from build123d import *

# Parameters (mm, degrees)
F1_DEPTH  = 7.5
F3_DEPTH  = 6
F5_DEPTH  = 3
F7_DEPTH  = 5
F8_W      = 24
F8_H      = 1.5
F9_DEPTH  = 3.75
F10_W     = 19
F10_H     = 2.5
F11_DEPTH = 9.7
F12_R     = 0.75
F13_DEPTH = 7.7
F14_W     = 24
F14_H     = 1.5
F15_DEPTH = 3.75
F16_DEPTH = 9.7


with BuildPart() as f1:
    # F0 (on Top) → F1 (new body)
    with BuildSketch(Plane.XY):
        with BuildLine():
            Line((-19.5, -14.9), (19.5, -14.9))
            ThreePointArc((19.5, -14.9), (20.9142135624, -14.3142135624), (21.5, -12.9))
            Line((21.5, -12.9), (21.5, 12.9))
            ThreePointArc((21.5, 12.9), (20.9142135624, 14.3142135624), (19.5, 14.9))
            Line((19.5, 14.9), (-19.5, 14.9))
            ThreePointArc((-19.5, 14.9), (-20.9142135624, 14.3142135624), (-21.5, 12.9))
            Line((-21.5, 12.9), (-21.5, -12.9))
            ThreePointArc((-21.5, -12.9), (-20.9142135624, -14.3142135624), (-19.5, -14.9))
        make_face()
    extrude(amount=F1_DEPTH)

    # F2 (on Top) → F3 (cut)
    with BuildSketch(Plane.XY):
        with BuildLine():
            Line((-13, -9.2), (13, -9.2))
            Line((13, -9.2), (13, -12.9))
            Line((13, -12.9), (17.5, -12.9))
            ThreePointArc((17.5, -12.9), (18.9142135624, -12.3142135624), (19.5, -10.9))
            Line((19.5, -10.9), (19.5, -7.5))
            Line((19.5, -7.5), (17.25, -7.5))
            Line((17.25, -7.5), (17.25, 7.5))
            Line((17.25, 7.5), (19.5, 7.5))
            Line((19.5, 7.5), (19.5, 10.9))
            ThreePointArc((19.5, 10.9), (18.9142135624, 12.3142135624), (17.5, 12.9))
            Line((17.5, 12.9), (13, 12.9))
            Line((13, 12.9), (13, 9.2))
            Line((13, 9.2), (-13, 9.2))
            Line((-13, 9.2), (-13, 12.9))
            Line((-13, 12.9), (-17.5, 12.9))
            ThreePointArc((-17.5, 12.9), (-18.9142135624, 12.3142135624), (-19.5, 10.9))
            Line((-19.5, 10.9), (-19.5, 7.5))
            Line((-19.5, 7.5), (-17.25, 7.5))
            Line((-17.25, 7.5), (-17.25, -7.5))
            Line((-17.25, -7.5), (-19.5, -7.5))
            Line((-19.5, -7.5), (-19.5, -10.9))
            ThreePointArc((-19.5, -10.9), (-18.9142135624, -12.3142135624), (-17.5, -12.9))
            Line((-17.5, -12.9), (-13, -12.9))
            Line((-13, -12.9), (-13, -9.2))
        make_face()
    extrude(amount=F3_DEPTH, mode=Mode.SUBTRACT)

    # F4 (on face) → F5 (join)
    with BuildSketch(Plane.XY.offset(7.5)):
        with BuildLine():
            Line((-16.5, -11.9), (16.5, -11.9))
            ThreePointArc((16.5, -11.9), (17.9142135624, -11.3142135624), (18.5, -9.9))
            Line((18.5, -9.9), (18.5, 9.9))
            ThreePointArc((18.5, 9.9), (17.9142135624, 11.3142135624), (16.5, 11.9))
            Line((16.5, 11.9), (-16.5, 11.9))
            ThreePointArc((-16.5, 11.9), (-17.9142135624, 11.3142135624), (-18.5, 9.9))
            Line((-18.5, 9.9), (-18.5, -9.9))
            ThreePointArc((-18.5, -9.9), (-17.9142135624, -11.3142135624), (-16.5, -11.9))
        make_face()
    extrude(amount=F5_DEPTH)

    # F6 (on face) → F7 (cut)
    with BuildSketch(Plane.XY.offset(10.5)):
        with BuildLine():
            Line((-15.75, -7.7), (15.75, -7.7))
            Line((15.75, -7.7), (15.75, -0.7749841599))
            Line((15.75, -0.7749841599), (16.4950450141, -0.7749841599))
            ThreePointArc((16.4950450141, -0.7749841599), (17.27499604, -0.0024775056), (16.5, 0.775))
            Line((16.5, 0.775), (15.75, 0.775))
            Line((15.75, 0.775), (15.75, 7.7))
            Line((15.75, 7.7), (-15.75, 7.7))
            Line((-15.75, 7.7), (-15.75, 0.7739160408))
            Line((-15.75, 0.7739160408), (-16.459024863, 0.7739160408))
            ThreePointArc((-16.459024863, 0.7739160408), (-17.2747289628, 0.020494736), (-16.5, -0.775))
            Line((-16.5, -0.775), (-15.75, -0.775))
            Line((-15.75, -0.775), (-15.75, -7.7))
        make_face()
    extrude(amount=-F7_DEPTH, mode=Mode.SUBTRACT)

    # F8 (on face) → F9 (cut)
    with BuildSketch(Plane(origin=(0, 0, 6), x_dir=(1, 0, 0), z_dir=(0, 0, -1))):
        with Locations((0, -8.45)):
            Rectangle(F8_W, F8_H)
    extrude(amount=-F9_DEPTH, mode=Mode.SUBTRACT)

    # F10 (on face) → F11 (cut)
    with BuildSketch(Plane(origin=(0, 0, 0), x_dir=(1, 0, 0), z_dir=(0, 0, -1))):
        with Locations((0, -10.45)):
            Rectangle(F10_W, F10_H)
    extrude(amount=-F11_DEPTH, mode=Mode.SUBTRACT)

    # F12 (on face) → F13 (cut)
    with BuildSketch(Plane(origin=(0, 0, 0), x_dir=(1, 0, 0), z_dir=(0, 0, -1))):
        with Locations((19.4, 0)):
            Circle(F12_R)
        with Locations((-19.4, 0)):
            Circle(F12_R)
    extrude(amount=-F13_DEPTH, mode=Mode.SUBTRACT)

    # F14 (on face) → F15 (cut)
    with BuildSketch(Plane(origin=(0, 0, 6), x_dir=(1, 0, 0), z_dir=(0, 0, -1))):
        with Locations((0, 8.45)):
            Rectangle(F14_W, F14_H)
    extrude(amount=-F15_DEPTH, mode=Mode.SUBTRACT)

    # F10 (on face) → F16 (cut)
    with BuildSketch(Plane(origin=(0, 0, 0), x_dir=(1, 0, 0), z_dir=(0, 0, -1))):
        with Locations((0, 10.45)):
            Rectangle(F10_W, F10_H)
    extrude(amount=-F16_DEPTH, mode=Mode.SUBTRACT)


solid = f1.part
Build history of the part. All positions in model axes, mm. A direction names the side the tool comes from. Give positions to 0.01 mm unless a question says otherwise; leave off trailing zeros. Order: outer loops, then holes, each group sorted by start corner. A loop starts at its lowest first (then second) coordinate and runs counter-clockwise, first axis right, second up. Notation, with made-up numbers: M 7.25,7 L 21.25,7 A15 ccw 21.25,25 Z; hole C 5,68.5 d9. An arc over 180 degrees is marked long. Put each result on its own line as item: value.
Item 1: Drop flat-ended pins along their axis: pin 1 Ø0.9 at (y, z) = (-4.5, 9) entering from +X; pin 2 Ø3 at (x, y) = (-6.5, -8) entering from -Z; pin 3 Ø0.6 at (x, z) = (-16, 9) entering from +Y. Give the stop position or say it passes through.
Results are:
pin 1: x = 18.5
pin 2: z = 9.7
pin 3: y = 11.9
Item 2: Cut at C-C on z = 1.5. Count the separate pieces of the cut face and the enclosed holes in it, then the cut area to 3 significant figures.
Results are:
separate pieces: 1
enclosed holes: 3
area: 437 mm2
Item 3: Cut at B-B on x = -4.5. Write the cut outline in (y, z).
Results are:
outline: M -14.9,0 L -11.7,0 L -11.7,9.7 L -9.2,9.7 L -9.2,9.75 L -7.7,9.75 L -7.7,10.5 L -11.9,10.5 L -11.9,7.5 L -14.9,7.5 Z; M 7.7,9.75 L 9.2,9.75 L 9.2,9.7 L 11.7,9.7 L 11.7,0 L 14.9,0 L 14.9,7.5 L 11.9,7.5 L 11.9,10.5 L 7.7,10.5 Z
Item 4: Wall check: probe 1 along X at (y, z) = (0, 4.5); probe 2 along X at (y, z) = (5.5, 5.5); probe 3 along Y at (x, z) = (2, 2.5). Give the ranges that are in metal, low to high.
Results are:
probe 1: -21.5 to -20.15, -18.65 to -17.25, 17.25 to 18.65, 20.15 to 21.5
probe 2: -21.5 to -17.25, 17.25 to 21.5
probe 3: -14.9 to -11.7, 11.7 to 14.9
Item 5: Which spindle directions (+Z, -Z, +X, -X, +Y, -Y) get a long thin tool onto all of the face, cutting with end or side? Do faces 5 (the face through (-19.5, 9, 3)), 6 (the face through (0, -7.7, 10)), 7 (the face through (0, 13, 7.5)). Say none if no direction does.
Results are:
face 5: -Z
face 6: +Z, -Z
face 7: +Z
Item 6: Cut at D-D on x = 12.5. Write the cut outline in (y, z), then the cut area to 3 significant figures.
Results are:
outline: M -14.9,0 L -9.2,0 L -9.2,6 L -7.7,6 L -7.7,10.5 L -11.9,10.5 L -11.9,7.5 L -14.9,7.5 Z; M 7.7,6 L 9.2,6 L 9.2,0 L 14.9,0 L 14.9,7.5 L 11.9,7.5 L 11.9,10.5 L 7.7,10.5 Z
area: 115 mm2
Item 7: Pull direction X, two halves, no side cores. Call faces 1 (the face through (-12, 8, 8)), 2 (the face through (0, 14.9, 4)), 3 (the face through (17.9, -11.33, 8.98)), 4 (the face through (-20.93, -14.3, 3.7)): +X half, -X half, draft (parallel to the pull), parting line (faces both ways), or undercut.
Results are:
face 1: undercut
face 2: draft
face 3: +X half
face 4: -X half
Item 8: Cut at A-A on y = 2.75. Write the cut outline in (x, z).
Results are:
outline: M -21.5,0 L -17.25,0 L -17.25,6 L -15.75,6 L -15.75,10.5 L -18.5,10.5 L -18.5,7.5 L -21.5,7.5 Z; M 15.75,6 L 17.25,6 L 17.25,0 L 21.5,0 L 21.5,7.5 L 18.5,7.5 L 18.5,10.5 L 15.75,10.5 Z
